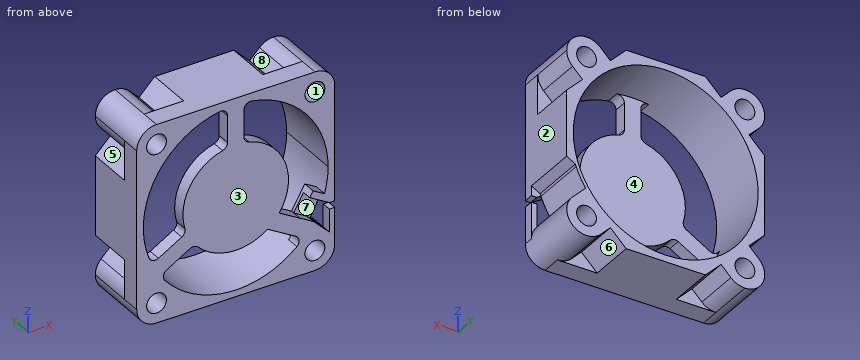
```python
from build123d import *

# Parameters (mm, degrees)
SKETCH2_W           = 30
SKETCH2_H           = 30
BOSS_EXTRUDE1_DEPTH = 10
SKETCH3_R           = 1.5
CUT_EXTRUDE1_DEPTH  = 24.452078799
CUT_EXTRUDE5_DEPTH  = 7
CIRPATTERN2_COUNT   = 4
BOSS_EXTRUDE2_START = -2
SKETCH5_R           = 8
BOSS_EXTRUDE2_DEPTH = 2
BOSS_EXTRUDE3_START = -2
BOSS_EXTRUDE3_DEPTH = 2
FILLET1_R           = 1
FILLET2_R           = 1
CUT_EXTRUDE8_DEPTH  = 1.5
CUT_EXTRUDE9_DEPTH  = 23.852789764


with BuildPart() as part:
    # Sketch2 → Boss-Extrude1 (new body)
    with BuildSketch(Plane(origin=(0, 0, 0), x_dir=(1, 0, 0), z_dir=(0, 1, 0))):
        Rectangle(SKETCH2_W, SKETCH2_H)
    extrude(amount=BOSS_EXTRUDE1_DEPTH)

    # Sketch3 → Cut-Extrude1 (cut, through all)
    with BuildSketch(Plane(origin=(0, 10, 0), x_dir=(1, 0, 0), z_dir=(0, 1, 0))):
        with BuildLine():
            ThreePointArc((9.626607334, 10.165059333), (-12.860258603, -5.532969245), (14, 0))
            ThreePointArc((14, 0), (13.005976139, 5.181175993), (10.165059333, 9.626607334))
            ThreePointArc((10.165059333, 9.626607334), (9.878679656, 9.878679656), (9.626607334, 10.165059333))
        make_face()
        with BuildLine():
            Line((15, 15), (12, 15))
            ThreePointArc((12, 15), (14.121320344, 14.121320344), (15, 12))
            Line((15, 12), (15, 15))
        make_face()
        with Locations(Location((12, 12, 0), (0, 0, 270))):
            Circle(SKETCH3_R)
    cut_extrude1 = extrude(amount=-CUT_EXTRUDE1_DEPTH, mode=Mode.SUBTRACT)

    # Sketch3<3> → Cut-Extrude5 (cut)
    with BuildSketch(Plane(origin=(0, 10, 0), x_dir=(1, 0, 0), z_dir=(0, 1, 0))):
        with BuildLine():
            Line((15, 6), (15, 12))
            ThreePointArc((15, 12), (14.771638598, 10.851949703), (14.121320344, 9.878679656))
            Line((14.121320344, 9.878679656), (12.621320344, 8.378679656))
            Line((12.621320344, 8.378679656), (15, 6))
        make_face()
        with BuildLine():
            Line((8.378679656, 12.621320344), (9.878679656, 14.121320344))
            ThreePointArc((9.878679656, 14.121320344), (10.851949703, 14.771638598), (12, 15))
            Line((12, 15), (6, 15))
            Line((6, 15), (8.378679656, 12.621320344))
        make_face()
    cut_extrude5 = extrude(amount=-CUT_EXTRUDE5_DEPTH, mode=Mode.SUBTRACT)

    # CirPattern2: Cut-Extrude1, Cut-Extrude5 ×4 about axis
    cirpattern2_axis = Axis((0, 0, 0), (0, 1, 0))
    add([cut_extrude1.rotate(cirpattern2_axis, i * 360 / CIRPATTERN2_COUNT) for i in range(1, CIRPATTERN2_COUNT)], mode=Mode.SUBTRACT)
    add([cut_extrude5.rotate(cirpattern2_axis, i * 360 / CIRPATTERN2_COUNT) for i in range(1, CIRPATTERN2_COUNT)], mode=Mode.SUBTRACT)

    # Sketch5 → Boss-Extrude2 (add)
    with BuildSketch(Plane.XZ.offset(BOSS_EXTRUDE2_START)):
        Circle(SKETCH5_R)
        with BuildLine():
            Line((-1.25, 7.901740315), (-1.25, 13.944084767))
            ThreePointArc((-1.25, 13.944084767), (0, 14), (1.25, 13.944084767))
            Line((1.25, 13.944084767), (1.25, 7.901740315))
            Line((1.25, 7.901740315), (-1.25, 7.901740315))
        make_face()
        with BuildLine():
            Line((-6.218107847, -5.033401912), (-11.450931641, -8.054574138))
            ThreePointArc((-11.450931641, -8.054574138), (-12.124355653, -7), (-12.700931641, -5.889510629))
            Line((-12.700931641, -5.889510629), (-7.468107847, -2.868338403))
            Line((-7.468107847, -2.868338403), (-6.218107847, -5.033401912))
        make_face()
        with BuildLine():
            Line((4.800907132, -6.399319551), (10.244405826, -9.542124987))
            ThreePointArc((10.244405826, -9.542124987), (11.062646674, -8.580084415), (11.790860146, -7.548219459))
            Line((11.790860146, -7.548219459), (6.585131773, -4.542690781))
            Line((6.585131773, -4.542690781), (4.800907132, -6.399319551))
        make_face()
    extrude(amount=BOSS_EXTRUDE2_DEPTH)

    # Sketch13 → Boss-Extrude3 (add)
    with BuildSketch(Plane.XZ.offset(BOSS_EXTRUDE3_START)):
        with BuildLine():
            Line((8.467510381, -8.516233923), (11.717510381, -2.887068799))
            Line((11.717510381, -2.887068799), (13.449561188, -3.887068799))
            ThreePointArc((13.449561188, -3.887068799), (12.179734535, -6.903192498), (10.244405826, -9.542124987))
            Line((10.244405826, -9.542124987), (8.467510381, -8.516233923))
        make_face()
    extrude(amount=BOSS_EXTRUDE3_DEPTH)

    # Fillet1
    # the kernel refuses this fillet: 1 mm, written as the material it adds along each edge
    with BuildSketch(Plane(origin=(10.244405826, 2, -9.542124987), x_dir=(-0.716571272890301, 0, -0.6975138786206146), z_dir=(0, -1, 0))) as fillet1_piece_1:
        with BuildLine():
            CenterArc((1.321230175, -0.998801992), FILLET1_R, 87.19514232, 108.576976785)
            Line((0.3588798, -1.270613979), (0, 0))
            ThreePointArc((0, 0), (0.685082313, 0.01677211), (1.370164625, 0))
        make_face()
    extrude(amount=2)
    with BuildSketch(Plane(origin=(-1.25, 2, 13.944084767), x_dir=(0, 0, -1), z_dir=(0, -1, 0)), Plane(origin=(-11.450931641, 2, -8.054574138), x_dir=(0.8660254037844306, 0, 0.5000000000000138), z_dir=(0, -1, 0))) as fillet1_piece_2:
        with BuildLine():
            CenterArc((1.14027674, -1), FILLET1_R, 90, 99.9667663)
            ThreePointArc((0.15536843, -1.173076923), (0.065284688, -0.58818072), (0, 0))
            Line((0, 0), (1.14027674, 0))
        make_face()
    extrude(amount=2)
    with BuildSketch(Plane(origin=(-12.700931641, 2, -5.889510629), x_dir=(0.8660254037844369, 0, 0.5000000000000029), z_dir=(0, -1, 0)), Plane(origin=(1.25, 2, 13.944084767), x_dir=(0, 0, -1), z_dir=(0, -1, 0))) as fillet1_piece_3:
        with BuildLine():
            CenterArc((1.14027674, 1), FILLET1_R, 170.0332337, 99.9667663)
            ThreePointArc((0.15536843, 1.173076923), (0.065284688, 0.58818072), (0, 0))
            Line((0, 0), (1.14027674, 0))
        make_face()
    extrude(amount=2)

    # Fillet2
    fillet2_edges = [part.edges().sort_by_distance(p)[0] for p in [
        (-7.468107847, 1, -2.868338403),
        (1.25, 1, 7.901740315),
        (-1.25, 1, 7.901740315),
        (-6.218107847, 1, -5.033401912),
    ]]
    fillet(fillet2_edges, radius=FILLET2_R)

    # Sketch9 → Cut-Extrude8 (cut)
    with BuildSketch(Plane.XZ):
        Polygon((9.717510381, -6.351170414), (11.790860146, -7.548219459), (12.621320344, -8.378679656), (14.121320344, -9.878679656), (14.2, -9.957359313), (14.2, -6.475035387), (15, -6.475035387), (15, -5.475035387), (14.2, -5.475035387), (11.217510381, -3.753094203), align=None)
    extrude(amount=-CUT_EXTRUDE8_DEPTH, mode=Mode.SUBTRACT)

    # Sketch10 → Cut-Extrude9 (cut, through all)
    with BuildSketch(Plane.XZ.offset(-1.5)):
        with BuildLine():
            ThreePointArc((13.569384529, -5.110949375), (12.93687053, -6.548845767), (12.152521667, -7.90988098))
            Line((12.152521667, -7.90988098), (14.121320344, -9.878679656))
            Line((14.121320344, -9.878679656), (14.2, -9.957359313))
            Line((14.2, -9.957359313), (14.2, -6.475035387))
            Line((14.2, -6.475035387), (15, -6.475035387))
            Line((15, -6.475035387), (15, -5.475035387))
            Line((15, -5.475035387), (14.2, -5.475035387))
            Line((14.2, -5.475035387), (13.569384529, -5.110949375))
        make_face()
        with BuildLine():
            ThreePointArc((13.693819896, -4.767525213), (13.632683665, -4.939629144), (13.569384529, -5.110949375))
            Line((13.569384529, -5.110949375), (14.2, -5.475035387))
            Line((14.2, -5.475035387), (15, -5.475035387))
            Line((15, -5.475035387), (15, -4))
            Line((15, -4), (13.693819896, -4.767525213))
        make_face()
        with BuildLine():
            Line((14.2, -9.957359313), (14.121320344, -9.878679656))
            ThreePointArc((14.121320344, -9.878679656), (14.771638598, -10.851949703), (15, -12))
            Line((15, -12), (15, -6.475035387))
            Line((15, -6.475035387), (14.2, -6.475035387))
            Line((14.2, -6.475035387), (14.2, -9.957359313))
        make_face()
    extrude(amount=-CUT_EXTRUDE9_DEPTH, mode=Mode.SUBTRACT)


solid = part.part
```
CAD build for the part. Positions are in the model's coordinates, mm. Face numbers are marked on the shaded views. A direction names the side the tool comes from. Give positions to 0.01 mm unless a question says otherwise; leave off trailing zeros. Loops run counter-clockwise (first coordinate to the right, second up) from the corner with the lowest first, then second, coordinate; pieces in that order, holes last. Notation, with made-up numbers: (52.5, 78.25) - (76.5, 78.25) arc R25 ccw to (76.5, 93.25) - close; hole circle Ø3 at (10, 48). An arc over 180 degrees is marked (long way). Put each result on its own line as item: value.
Q1. Tool access for the marked faces 4, 5, 6, 7 and 8: list every direction of +Z, -Z, +X, -X, +Y, -Y with a clear straight run to the whole face (end or side of a thin tool).
Filled in:
face 4: +Y
face 5: -X, +Y
face 6: -Z, +Y
face 7: -Y
face 8: +Z, +Y
Q2. Slice it at B-B (z = 3). Give the cut face in (x, y), plus the area to 3 significant figures.
Filled in:
outline: (-15, 0) - (-13.67, 0) - (-13.67, 10) - (-15, 10) - close; (-7.42, 0) - (7.42, 0) - (7.42, 2) - (-7.42, 2) - close; (13.67, 0) - (15, 0) - (15, 10) - (13.67, 10) - close
area: 56.2 mm²
Q3. Slice it at D-D (y = 9.5). Give the number of separate pieces and of enclosed holes in the cut face, plus the area to 3 significant figures.
Filled in:
separate pieces: 1
enclosed holes: 5
area: 196 mm²
Q4. Mould opens along X. For the marked faces 1, 2 and 3 say: pulls with the +X half, pulls with the -X half, needs draft (parallel to the pull), parting line crosses it, or undercut.
Filled in:
face 1: undercut
face 2: pulls with the +X half
face 3: needs draft
Q5. Slice it at C-C (x = 13). Give the cut face in (y, z).
Filled in:
outline: (0, -14.83) - (10, -14.83) - (10, -13.12) - (0, -13.12) - close; (0, -10.88) - (10, -10.88) - (10, -8.76) - (0, -8.76) - close; (0, -4.78) - (1.5, -4.78) - (1.5, -6.42) - (10, -6.42) - (10, -5.2) - (2, -5.2) - (2, -3.63) - (0, -3.63) - close; (0, 5.2) - (10, 5.2) - (10, 8) - (3, 8) - (3, 8.76) - (10, 8.76) - (10, 10.88) - (0, 10.88) - close; (0, 13.12) - (10, 13.12) - (10, 14.83) - (0, 14.83) - close
Q6. Slice it at A-A (x = 0). Give the cut face in (y, z), plus the area to 3 significant figures.
Filled in:
outline: (0, -15) - (10, -15) - (10, -14) - (0, -14) - close; (0, -8) - (2, -8) - (2, 14) - (10, 14) - (10, 15) - (0, 15) - close
area: 64.0 mm²
Q7. Probe line 1 along Z through (x, y) = (0, 5.25); line 2 along Z through (x, y) = (11.5, 8.75); line 3 along Y through (x, z) = (-7.25, -3). List the from-to ranges inside material, lowest first.
Filled in:
line 1: z = -15 to -14, 14 to 15
line 2: z = -14.96 to -13.41, -10.59 to -7.98, 7.98 to 10.59, 13.41 to 14.96
line 3: y = 0 to 2
Q8. Flat gauge pins, fed straight in: pin 1 (3 mm diameter, centred on x = -6.5, z = -10, fed in from -Y); pin 2 (2.5 mm diameter, centred on x = -14, z = 9.5, fed in from +Y); pin 3 (1.1 mm diameter, centred on x = 14.5, z = -5, fed in from +Y); pin 4 (1.5 mm diameter, centred on y = 8, z = 8.5, fed in from -X). Where does each tip first touch, or does it go through?
Filled in:
pin 1: passes through
pin 2: stops at y = 10
pin 3: stops at y = 1.5
pin 4: stops at x = -13.49
